```python
from build123d import *

# Parameters (mm, degrees)
BOSS_EXTRUDE1_DEPTH = 3
CUT_EXTRUDE2_DEPTH  = 10


with BuildPart() as part:
    # Sketch1 → Boss-Extrude1 (new body)
    with BuildSketch(Plane.XY):
        with BuildLine():
            Line((0, 29), (52, 29))
            ThreePointArc((52, 29), (56.242640687, 27.242640687), (58, 23))
            Line((58, 23), (58, 0))
            Line((58, 0), (0, 0))
            Line((0, 0), (0, 29))
        make_face()
    extrude(amount=BOSS_EXTRUDE1_DEPTH)

    # Sketch4 → Cut-Extrude2 (cut)
    with BuildSketch(Plane.XY.offset(3)):
        with BuildLine():
            Line((10, 15), (48, 15))
            ThreePointArc((48, 15), (52, 11), (48, 7))
            Line((48, 7), (10, 7))
            ThreePointArc((10, 7), (6, 11), (10, 15))
        make_face()
    extrude(amount=-CUT_EXTRUDE2_DEPTH, mode=Mode.SUBTRACT)


solid = part.part
```
Model file for the job. Use its own axes, mm. A direction names the side the tool comes from. Coordinates: 2 decimals unless noted, no trailing zeros. Write each loop counter-clockwise with the first axis right and the second up, starting at its lowest first coordinate (ties: lowest second). Pieces come first, ordered by that corner, then holes. Notation, with made-up numbers: (66, 20.5) - (105, 20.5) arc R16 cw to (105, 38.5) - close; hole circle Ø1 at (35.5, 63.25). An arc over 180 degrees is marked (long way). One line per item, written item: value. Start each with the question number.
1. Tool access for faces 1 (the cylindrical face through (6, 11, 2)), 2 (the flat face through (29, 0, 1)): list every direction of +Z, -Z, +X, -X, +Y, -Y with a clear straight run to the whole face (end or side of a thin tool).
2. Slice it at A-A (x = 34). Write the cut outline in (y, z).
3. Probe line 1 (Y direction, x = 28.5, z = 1.7); line 2 (X direction, y = 11.25, z = 0.45); line 3 (Y direction, x = 49.5, z = 0.7). List the from-to ranges inside material, lowest first. Write a range as from..to.
4. Slice it at C-C (z = 1.75). Write the cut outline in (x, y), plus the area to 3 significant figures.
5. Mould opens along X. For faces 3 (the cylindrical face through (56.196, 27.289, 1.479)), 4 (the flat face through (29, 7, 2)), 5 (the flat face through (29, 18, 0)), 6 (the flat face through (29, 15, 2)) say: released by +X, released by -X, zero draft, split by the parting line, or undercut.
6. Slice it at B-B (y = 11). Write the cut outline in (x, z).
Answers below:
1. face 1: +Z, -Z
1. face 2: +Z, -Z, +X, -X, -Y
2. outline: (0, 0) - (7, 0) - (7, 3) - (0, 3) - close; (15, 0) - (29, 0) - (29, 3) - (15, 3) - close
3. line 1: y = 0..7, 15..29
3. line 2: x = 0..6.01, 51.99..58
3. line 3: y = 0..7.29, 14.71..29
4. outline: (0, 0) - (58, 0) - (58, 23) arc R6 ccw to (52, 29) - (0, 29) - close; hole (10, 7) - (48, 7) arc R4 ccw to (48, 15) - (10, 15) arc R4 ccw to start
4. area: 1,320 mm^2
5. face 3: released by +X
5. face 4: undercut
5. face 5: zero draft
5. face 6: undercut
6. outline: (0, 0) - (6, 0) - (6, 3) - (0, 3) - close; (52, 0) - (58, 0) - (58, 3) - (52, 3) - close
